from build123d import *

# Parameters (mm, degrees)
SKETCH1_W               = 533.4
SKETCH1_H               = 152.4
BOSS_EXTRUDE1_DEPTH     = 6.35
SKETCH2_W               = 107.95
SKETCH2_H               = 6.35
CUT_EXTRUDE2_DEPTH      = 7.35
LPATTERN1_COUNT         = 3
LPATTERN1_PITCH         = 133.35
LPATTERN1_COL_COUNT     = 3
LPATTERN1_COL_PITCH     = 133.35
MIRROR2_COPY_1_SKETCH_W = 107.95
MIRROR2_COPY_1_SKETCH_H = 6.35
MIRROR2_COPY_1_DEPTH    = 7.35
MIRROR2_COPY_2_SKETCH_W = 107.95
MIRROR2_COPY_2_SKETCH_H = 6.35
MIRROR2_COPY_2_DEPTH    = 7.35
MIRROR2_COPY_3_SKETCH_W = 107.95
MIRROR2_COPY_3_SKETCH_H = 6.35
MIRROR2_COPY_3_DEPTH    = 7.35
MIRROR2_COPY_4_SKETCH_W = 107.95
MIRROR2_COPY_4_SKETCH_H = 6.35
MIRROR2_COPY_4_DEPTH    = 7.35


with BuildPart() as part:
    # Sketch1 → Boss-Extrude1 (new body)
    with BuildSketch(Plane(origin=(0, 0, 0), x_dir=(1, 0, 0), z_dir=(0, 1, 0))):
        Rectangle(SKETCH1_W, SKETCH1_H)
    extrude(amount=BOSS_EXTRUDE1_DEPTH)

    # Sketch2 → Cut-Extrude2 (cut, through all)
    with BuildSketch(Plane(origin=(0, 6.35, 0), x_dir=(1, 0, 0), z_dir=(0, 1, 0))):
        with Locations((0, -73.025)):
            Rectangle(SKETCH2_W, SKETCH2_H)
    cut_extrude2 = extrude(amount=-CUT_EXTRUDE2_DEPTH, mode=Mode.SUBTRACT)

    # LPattern1: Cut-Extrude2 ×3
    with Locations(*[(-i * LPATTERN1_PITCH, 0, 0) for i in range(1, LPATTERN1_COUNT)]):
        add(cut_extrude2, mode=Mode.SUBTRACT)

    # LPattern1 col: Cut-Extrude2 ×3
    with Locations(*[(i * LPATTERN1_COL_PITCH, 0, 0) for i in range(1, LPATTERN1_COL_COUNT)]):
        add(cut_extrude2, mode=Mode.SUBTRACT)

    # Mirror2: Cut-Extrude2 across plane
    add(cut_extrude2.mirror(Plane.XY), mode=Mode.SUBTRACT)

    # Mirror2 copy 1 sketch → Mirror2 copy 1 (cut, through all)
    with BuildSketch(Plane(origin=(-133.35, 6.35, 0), x_dir=(1, 0, 0), z_dir=(0, 1, 0))):
        with Locations((0, 73.025)):
            Rectangle(MIRROR2_COPY_1_SKETCH_W, MIRROR2_COPY_1_SKETCH_H)
    extrude(amount=-MIRROR2_COPY_1_DEPTH, mode=Mode.SUBTRACT)

    # Mirror2 copy 2 sketch → Mirror2 copy 2 (cut, through all)
    with BuildSketch(Plane(origin=(-266.7, 6.35, 0), x_dir=(1, 0, 0), z_dir=(0, 1, 0))):
        with Locations((0, 73.025)):
            Rectangle(MIRROR2_COPY_2_SKETCH_W, MIRROR2_COPY_2_SKETCH_H)
    extrude(amount=-MIRROR2_COPY_2_DEPTH, mode=Mode.SUBTRACT)

    # Mirror2 copy 3 sketch → Mirror2 copy 3 (cut, through all)
    with BuildSketch(Plane(origin=(133.35, 6.35, 0), x_dir=(1, 0, 0), z_dir=(0, 1, 0))):
        with Locations((0, 73.025)):
            Rectangle(MIRROR2_COPY_3_SKETCH_W, MIRROR2_COPY_3_SKETCH_H)
    extrude(amount=-MIRROR2_COPY_3_DEPTH, mode=Mode.SUBTRACT)

    # Mirror2 copy 4 sketch → Mirror2 copy 4 (cut, through all)
    with BuildSketch(Plane(origin=(266.7, 6.35, 0), x_dir=(1, 0, 0), z_dir=(0, 1, 0))):
        with Locations((0, 73.025)):
            Rectangle(MIRROR2_COPY_4_SKETCH_W, MIRROR2_COPY_4_SKETCH_H)
    extrude(amount=-MIRROR2_COPY_4_DEPTH, mode=Mode.SUBTRACT)


solid = part.part
Check sheet for the modelled part. Datum: model origin and axes. Units: mm. Round coordinates to 2 decimals unless told otherwise and drop trailing zeros. Order: outer loops, then holes, each group sorted by start corner. A loop starts at its lowest first (then second) coordinate and runs counter-clockwise, first axis right, second up.
Q1. Depth check by flat-ended pin: P1, Ø3, axis at x = 143, y = 3, coming from the -Z side; P2, Ø3, axis at x = -228, y = 5, coming from the +Z side; P3, Ø1.9, axis at y = 2, z = 73.5, coming from the +X side (3 decimals). Enter the tip coordinate at first touch or a pass-through.
Filled sheet:
P1: stops at z = -69.85
P2: stops at z = 69.85
P3: stops at x = 212.725
Q2. Scan line: L1, parallel to Z at x = -123, y = 3.5. Record every from-to range of solid material in increasing order.
Filled sheet:
L1: z = -69.85 to 69.85
Q3. Cross-section at A-A, the plane x = 131. Enter the section's corners in (y, z), plus the area to 3 significant figures.
Filled sheet:
outline: (0, -69.85) - (6.35, -69.85) - (6.35, 69.85) - (0, 69.85) - close
area: 887 mm2
